Verification items for this drawing (mm, ordinates from the low corner). A direction names the side the tool comes from. Coordinates: 2 decimals unless noted, no trailing zeros. Order: outer loops, then holes, each group sorted by start corner. A loop starts at its lowest first (then second) coordinate and runs counter-clockwise, first axis right, second up. Notation, with made-up numbers: M -37,48 L -32,48 A28 cw -32,69 Z; hole C 9,-34.5 d4. An arc over 180 degrees is marked long. Answer as a JSON object with one key per item and string values. Group by question number.
(1) Cross-section at B-B (x = 40.5). Enter the section's corners in (y, z), plus the area to 3 significant figures.
(2) Cross-section at C-C (y = 0.75). Count the separate pieces of the cut face and the enclosed holes in it, plus the area to 3 significant figures.
(3) Cross-section at D-D (x = 19.5). Enter the section's corners in (y, z).
(4) Material ranges on line 1 (Z direction, x = 41.5, y = 5); line 2 (X direction, y = 3.75, z = 57) (1 decimal); line 3 (Z direction, x = 43.5, y = 7.75), recorded low to high.
(5) Access from +Z, -Z, +X, -X, +Y, -Y to the whole of each face (thin tool, end or side, straight path). Record for the marked faces 4 and 5.
(6) Cross-section at A-A (x = 33). Enter the section's corners in (y, z).
(7) Mould release check, pull along X, two halves, no side actions. Record for the marked faces 1, 2 and 3: released by +X, released by -X, zero draft, split by the parting line, or undercut.
(8) Gauge pin test, flat end, axial feed: pin 1 Ø5 at (x, y) = (11.5, 3) entering from -Z. Record the tip position at first contact, or that the pin passes through.
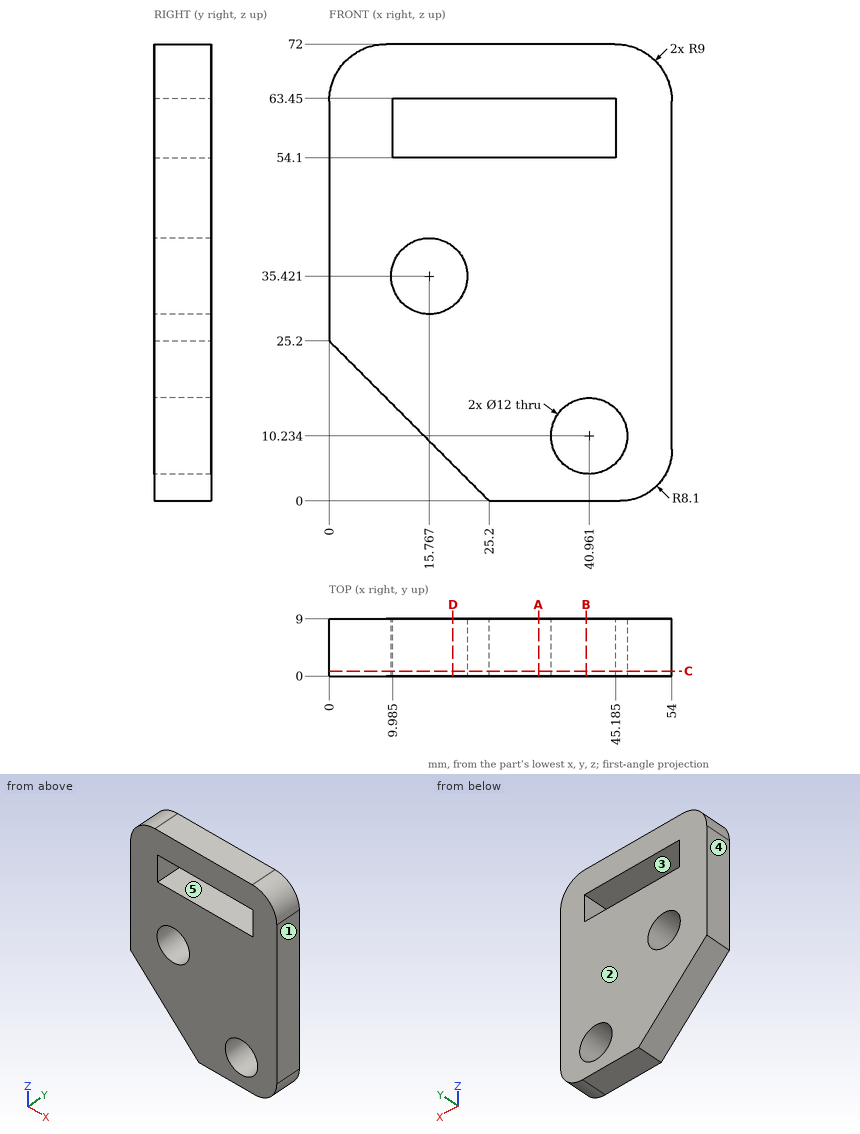
Taken from the geometry:
{
 "1": {"outline": "M 0,0 L 9,0 L 9,4.25 L 0,4.25 Z; M 0,16.22 L 9,16.22 L 9,54.1 L 0,54.1 Z; M 0,63.45 L 9,63.45 L 9,72 L 0,72 Z", "area": "456 mm²"},
 "2": {"separate pieces": "1", "enclosed holes": "3", "area": "2,970 mm²"},
 "3": {"outline": "M 0,5.7 L 9,5.7 L 9,30.72 L 0,30.72 Z; M 0,40.12 L 9,40.12 L 9,54.1 L 0,54.1 Z; M 0,63.45 L 9,63.45 L 9,72 L 0,72 Z"},
 "4": {"line 1": "z = 0 to 4.26, 16.21 to 54.1, 63.45 to 72", "line 2": "x = 0 to 10, 45.2 to 54", "line 3": "z = 0 to 4.8, 15.67 to 54.1, 63.45 to 72"},
 "5": {"face 4": "+Z, -Z, -X, +Y, -Y", "face 5": "+Y, -Y"},
 "6": {"outline": "M 0,0 L 9,0 L 9,54.1 L 0,54.1 Z; M 0,63.45 L 9,63.45 L 9,72 L 0,72 Z"},
 "7": {"face 1": "released by +X", "face 2": "zero draft", "face 3": "undercut"},
 "8": {"pin 1": "stops at z = 11.2"}
}
